from build123d import *

# Parameters (mm, degrees)
SKETCH1_W                        = 152.4
SKETCH1_H                        = 76.2
BOSS_EXTRUDE1_DEPTH              = 6.35
F_17_64_0_26563_DIAMETER_HOLE1_D = 6.747002
LPATTERN1_COUNT                  = 4
LPATTERN1_PITCH                  = 38.1
LPATTERN1_COUNT_DIR2             = 2
LPATTERN1_PITCH_DIR2             = 38.1


with BuildPart() as part:
    # Sketch1 → Boss-Extrude1 (new body)
    with BuildSketch(Plane.XY):
        with Locations((76.2, 38.1)):
            Rectangle(SKETCH1_W, SKETCH1_H)
    extrude(amount=BOSS_EXTRUDE1_DEPTH)

    # 17/64 (0.26563) Diameter Hole1 (through all)
    with Locations(Plane.XY.offset(6.35)):
        with Locations((19.05, 19.05)):
            f_17_64_0_26563_diameter_hole1 = Hole(F_17_64_0_26563_DIAMETER_HOLE1_D / 2)

    # LPattern1: 17_64 _0.26563_ Diameter Hole1 4 × 2
    with Locations(*[(i * LPATTERN1_PITCH, j * LPATTERN1_PITCH_DIR2, 0) for i in range(LPATTERN1_COUNT) for j in range(LPATTERN1_COUNT_DIR2) if (i, j) != (0, 0)]):
        add(f_17_64_0_26563_diameter_hole1, mode=Mode.SUBTRACT)


solid = part.part
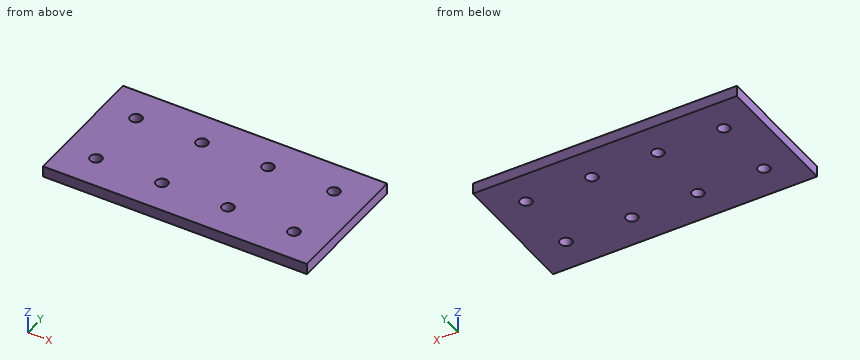
Part model, mm, in its own coordinate system. Give positions to 0.01 mm unless a question says otherwise; leave off trailing zeros. Loops run counter-clockwise (first coordinate to the right, second up) from the corner with the lowest first, then second, coordinate; pieces in that order, holes last. Notation, with made-up numbers: M -13,69 L 29,69 A34 ccw 29,103 Z; hole C 56,14 d11. An arc over 180 degrees is marked long. Put each result on its own line as item: value. Start each with the question number.
1) Saw through at A-A (y = 19.05). List the corners of the cut face in (x, z).
2) Saw through at B-B (z = 2). State how many separate pieces and enclosed holes the cut face has, then the cut area to 3 significant figures.
3) Saw through at C-C (x = 57.15). List the corners of the cut face in (y, z).
4) Probe probe 1 along Y at (x, z) = (57.15, 4.25); probe 2 along Y at (x, z) = (21.5, 5.5); probe 3 along X at (y, z) = (21, 5.75). List the from-to ranges inside material, lowest first.
5) Flat gauge pin, fed straight in: pin 1 (11 mm diameter, centred on x = 95.25, y = 57.15, fed in from -Z). Where does the tip first touch, or does it go through?
Numbers:
1. outline: M 0,0 L 15.68,0 L 15.68,6.35 L 0,6.35 Z; M 22.42,0 L 53.78,0 L 53.78,6.35 L 22.42,6.35 Z; M 60.52,0 L 91.88,0 L 91.88,6.35 L 60.52,6.35 Z; M 98.62,0 L 129.98,0 L 129.98,6.35 L 98.62,6.35 Z; M 136.72,0 L 152.4,0 L 152.4,6.35 L 136.72,6.35 Z
2. separate pieces: 1
2. enclosed holes: 8
2. area: 11,300 mm^2
3. outline: M 0,0 L 15.68,0 L 15.68,6.35 L 0,6.35 Z; M 22.42,0 L 53.78,0 L 53.78,6.35 L 22.42,6.35 Z; M 60.52,0 L 76.2,0 L 76.2,6.35 L 60.52,6.35 Z
4. probe 1: 0 to 15.68, 22.42 to 53.78, 60.52 to 76.2
4. probe 2: 0 to 16.73, 21.37 to 54.83, 59.47 to 76.2
4. probe 3: 0 to 16.3, 21.8 to 54.4, 59.9 to 92.5, 98 to 130.6, 136.1 to 152.4
5. pin 1: z = 0
